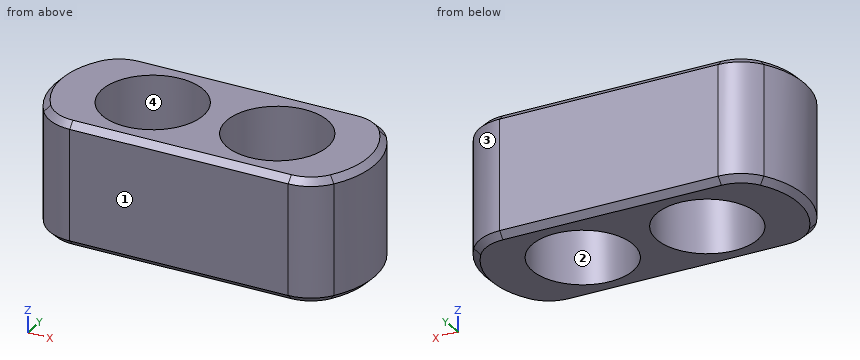
Solid Edge part; units mm, degrees
sketch "Sketch1" plane through (0, 0, 0) normal (0, 0, 1) x (1, 0, 0)
  arc A0 (20.4574, 11) -> (20.4574, -11) centre (11.7971, 0) cw
  line L0 (-20.4574, -11) -> (20.4574, -11)
  arc A1 (-20.4574, 11) -> (-20.4574, -11) centre (-11.7971, 0) ccw
  line L1 (-20.4574, 11) -> (20.4574, 11)
extrude "Ajout_matière_1" add sketch "Sketch1" against normal blind 20
sketch "Sketch2" plane through (0, 0, 0) normal (0, 0, 1) x (-1, 0, 0)
  circle A0 centre (-10, 0) radius 8.2
  circle A1 centre (10, 0) radius 8.2
extrude "Cutout1" cut sketch "Sketch2" against normal through all and the other way up to next
fillet "Congé_1" radius 7 4 edges at (20.4574, -11, -10) (20.4574, 11, -10) (-20.4574, 11, -10) (-20.4574, -11, -10)
chamfer "Chanfrein_1" distance 1 angle 45 16 edges at (0, -11, 0) (-20.782, -10.2048, 0) (-25.7971, 0, 0) (-20.782, 10.2048, 0) (0, 11, 0) (20.782, 10.2048, 0) (25.7971, 0, 0) (20.782, -10.2048, 0) (0, -11, -20) (-20.782, -10.2048, -20) (-25.7971, 0, -20) (-20.782, 10.2048, -20) (0, 11, -20) (20.782, 10.2048, -20) (25.7971, 0, -20) (20.782, -10.2048, -20)
properties material "Plastique ABS, haute performance"
Verification items for the finished model (mm, model axes). Face numbers are marked on the shaded views. Coordinates: 2 decimals unless noted, no trailing zeros. Loops run counter-clockwise (first coordinate to the right, second up) from the corner with the lowest first, then second, coordinate; pieces in that order, holes last. Notation, with made-up numbers: (68.5, -1.5) -> (97.5, -1.5) arc R30 cw to (97.5, 36.5) -> close; hole circle Ø5 at (45, -15). An arc over 180 degrees is marked (long way). Answer in a Markdown table with one row per item. Add a question column.
1. Material ranges on probe 1 along X at (y, z) = (0, -6); probe 2 along Y at (x, z) = (-10, -8.25); probe 3 along X at (y, z) = (1.5, -4.75), recorded low to high. Write a range as [from, to].
2. Depth check by flat-ended pin: P1, Ø10, axis at y = -5.5, z = -12, coming from the +X side; P2, Ø10, axis at x = 10, y = 0, coming from the +Z side; P3, Ø2, axis at y = 4.5, z = -2.5, coming from the -X side; P4, Ø2, axis at y = 2.5, z = -8, coming from the +X side. Enter the tip coordinate at first touch or a pass-through.
3. Section check B-B, the plane y = 0. Enter the section's corners in (x, z).
4. Section check C-C, the plane z = -10. Enter the section's corners in (x, y), then the cut area to 3 significant figures.
5. Section check A-A, the plane x = 10. Enter the section's corners in (y, z), then the cut area to 3 significant figures.
6. Section check D-D, the plane y = 6.5. Give the number of separate pieces and of enclosed holes in the cut face, then the cut area to 3 significant figures.
7. Draft check along X on the marked faces 1, 2, 3 and 4. Enter one of: +X half, -X half, draft (parallel to the pull), parting line (faces both ways), or undercut.
Derived:
| question | item | result |
|---|---|---|
| 1 | probe 1 | x = [-25.8, -18.2], [-1.8, 1.8], [18.2, 25.8] |
| 1 | probe 2 | y = [-11, -8.2], [8.2, 11] |
| 1 | probe 3 | x = [-25.72, -18.06], [-1.94, 1.94], [18.06, 25.72] |
| 2 | P1 | stops at x = 25.79 |
| 2 | P2 | passes through |
| 2 | P3 | stops at x = -25.35 |
| 2 | P4 | stops at x = 25.72 |
| 3 | outline | (-25.8, -19) -> (-24.8, -20) -> (-18.2, -20) -> (-18.2, 0) -> (-24.8, 0) -> (-25.8, -1) -> close; (-1.8, -20) -> (1.8, -20) -> (1.8, 0) -> (-1.8, 0) -> close; (18.2, -20) -> (24.8, -20) -> (25.8, -19) -> (25.8, -1) -> (24.8, 0) -> (18.2, 0) -> close |
| 4 | outline | (-23.29, -8) arc R7 ccw to (-17.54, -11) -> (17.54, -11) arc R7 ccw to (23.29, -8) arc R14 ccw to (23.29, 8) arc R7 ccw to (17.54, 11) -> (-17.54, 11) arc R7 ccw to (-23.29, 8) arc R14 ccw to start; hole circle Ø16.4 at (-10, 0); hole circle Ø16.4 at (10, 0) |
| 4 | area | 636 mm² |
| 5 | outline | (-11, -19) -> (-10, -20) -> (-8.2, -20) -> (-8.2, 0) -> (-10, 0) -> (-11, -1) -> close; (8.2, -20) -> (10, -20) -> (11, -19) -> (11, -1) -> (10, 0) -> (8.2, 0) -> close |
| 5 | area | 110 mm² |
| 6 | separate pieces | 3 |
| 6 | enclosed holes | 0 |
| 6 | area | 566 mm² |
| 7 | face 1 | draft |
| 7 | face 2 | undercut |
| 7 | face 3 | +X half |
| 7 | face 4 | undercut |
